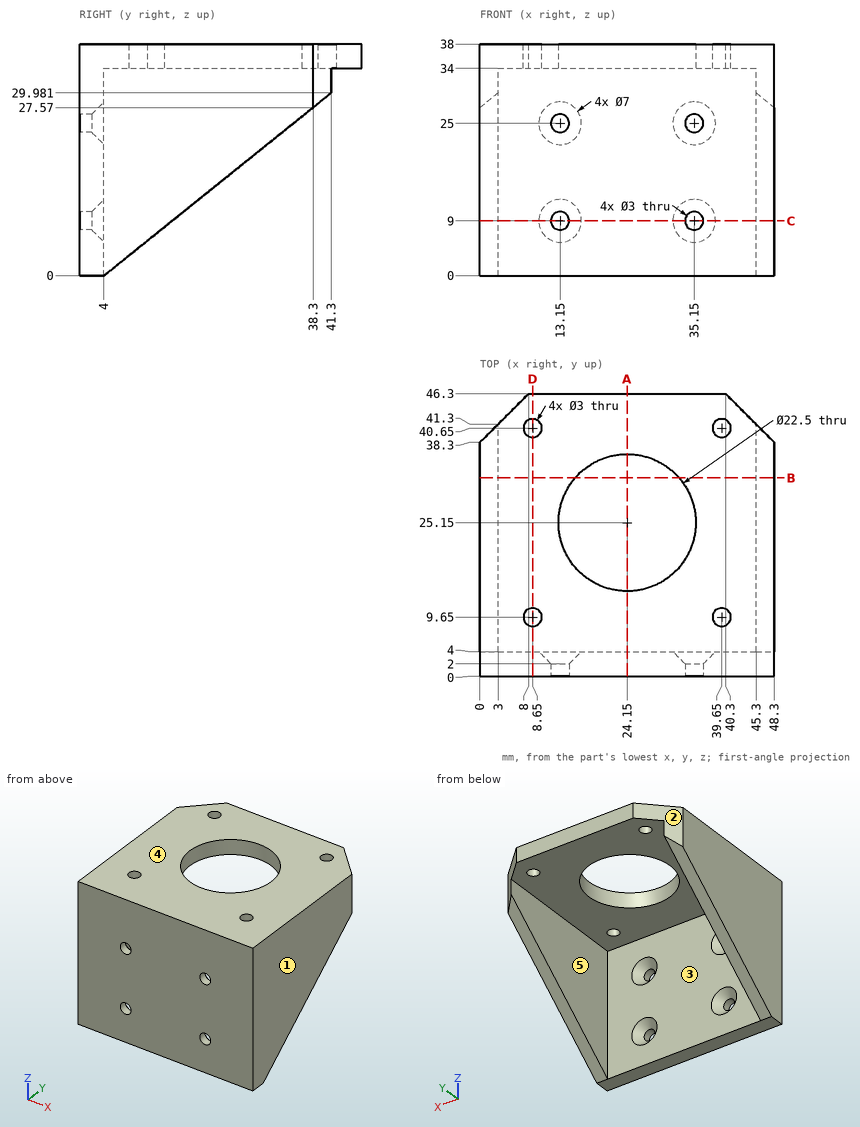
Here's the drawing with two shaded views (mm, measured from the low corner). I have some questions. A direction names the side the tool comes from. Round coordinates to 2 decimals unless told otherwise and drop trailing zeros. Order: outer loops, then holes, each group sorted by start corner. A loop starts at its lowest first (then second) coordinate and runs counter-clockwise, first axis right, second up. Notation, with made-up numbers: (53, -5.5) -> (79, -5.5) arc R24 ccw to (79, 22.5) -> close; hole circle Ø1 at (-32.75, 76.25). An arc over 180 degrees is marked (long way). Return JSON: item names as keys, results as strings.
Q1. If we section it at C-C on z = 9: List the corners of the cut face in (x, y) for me, plus the area to 3 significant figures.
Filled sheet:
{"outline": "(0, 0) -> (11.65, 0) -> (11.65, 2) -> (9.65, 4) -> (3, 4) -> (3, 15.2) -> (0, 15.2) -> close; (14.65, 0) -> (33.65, 0) -> (33.65, 2) -> (31.65, 4) -> (16.65, 4) -> (14.65, 2) -> close; (36.65, 0) -> (48.3, 0) -> (48.3, 15.2) -> (45.3, 15.2) -> (45.3, 4) -> (38.65, 4) -> (36.65, 2) -> close", "area": "228 mm^2"}
Q2. If we mould it in two halves opening along X, with no side actions, what happens to the marked faces 1, 2 and 3? For each: released by +X, released by -X, zero draft, split by the parting line, or undercut.
Filled sheet:
{"face 1": "released by +X", "face 2": "released by -X", "face 3": "undercut"}
Q3. I need wall thicknesses on line 1 along X through (y, z) = (18.5, 19); line 2 along X through (y, z) = (1, 9); line 3 along X through (y, z) = (40.65, 35.65). Which ranges of each line are inside material? Lowest first, please. Write a range as from..to.
Filled sheet:
{"line 1": "x = 0..3, 45.3..48.3", "line 2": "x = 0..11.65, 14.65..33.65, 36.65..48.3", "line 3": "x = 2.35..7.15, 10.15..38.15, 41.15..45.95"}
Q4. For pin 1 Ø4 at (x, y) = (7, 5) entering from -Z; pin 2 Ø4 at (x, y) = (8.65, 40.65) entering from -Z; pin 3 Ø2.5 at (x, z) = (35.15, 9) entering from -Y; pin 4 Ø5 at (x, z) = (26, 21.5) entering from +Y, each with a flat end and sliding along its axis, tell me the tip position at first contact or that it passes through.
Filled sheet:
{"pin 1": "stops at z = 0", "pin 2": "stops at z = 34", "pin 3": "passes through", "pin 4": "stops at y = 4"}
Q5. If we section it at A-A on x = 24.15: List the corners of the cut face in (y, z) for me.
Filled sheet:
{"outline": "(0, 0) -> (4, 0) -> (4, 34) -> (13.9, 34) -> (13.9, 38) -> (0, 38) -> close; (36.4, 34) -> (46.3, 34) -> (46.3, 38) -> (36.4, 38) -> close"}
Q6. If we section it at D-D on x = 8.65: List the corners of the cut face in (y, z) for me, plus the area to 3 significant figures.
Filled sheet:
{"outline": "(0, 0) -> (4, 0) -> (4, 34) -> (8.15, 34) -> (8.15, 38) -> (0, 38) -> close; (11.15, 34) -> (39.15, 34) -> (39.15, 38) -> (11.15, 38) -> close; (42.15, 34) -> (46.3, 34) -> (46.3, 38) -> (42.15, 38) -> close", "area": "297 mm^2"}
Q7. If we section it at B-B on y = 32.5: List the corners of the cut face in (x, z) for me, plus the area to 3 significant figures.
Filled sheet:
{"outline": "(0, 22.91) -> (3, 22.91) -> (3, 34) -> (15.63, 34) -> (15.63, 38) -> (0, 38) -> close; (32.67, 34) -> (45.3, 34) -> (45.3, 22.91) -> (48.3, 22.91) -> (48.3, 38) -> (32.67, 38) -> close", "area": "192 mm^2"}
Q8. Which directions (+Z, -Z, +X, -X, +Y, -Y) give clear straight access to the entire face, cutting with the end or side of a thin tool? Please do the marked faces 4 and 5.
Filled sheet:
{"face 4": "+Z, +X, -X, +Y, -Y", "face 5": "-Z, +Y"}
